Autodesk Inventor part; units mm, degrees
ref_plane "a1_XY" through (0, 8.636, -14.224) normal (0, 1, 0) x (1, 0, 0)
ref_plane "a1_YZ" through (0, 8.636, -14.224) normal (1, 0, 0) x (0, 0, -1)
ref_plane "a1_ZX" through (0, 8.636, -14.224) normal (0, 0, -1) x (0, 1, 0)
sketch "Sketch_1" plane through (0, 0, 0) normal (0, 0, 1) x (1, 0, 0)
  line L0 (0, 0) -> (0, 8.636)
  line L1 (0, 8.636) -> (14.224, 8.636)
  line L2 (14.224, 8.636) -> (14.224, 0)
  line L3 (14.224, 0) -> (0, 0)
  line L4 (0, 0) -> (0, 8.636)
revolve "Revolution1" add sketch "Sketch_1" angle 360 about axis through (0, 0, 0) along (0, -1, 0)
sketch "Sketch_37" plane through (0, 0, 0) normal (0, 0, 1) x (1, 0, 0)
  line L0 (-5.9667, 5.08) -> (-14.224, 5.08)
  line L1 (-14.224, 5.08) -> (-14.224, 9.0488)
  line L2 (-14.224, 9.0488) -> (-13.716, 9.0488)
  line L3 (-13.716, 9.0488) -> (-13.716, 7.493)
  line L4 (-13.716, 7.493) -> (-13.2867, 7.0637)
  line L5 (-13.2867, 7.0637) -> (-7.112, 7.0637)
  line L6 (-7.112, 7.0637) -> (-5.9667, 5.08)
  line L7 (-5.9667, 5.08) -> (-14.224, 5.08)
revolve "Revolution2" cut sketch "Sketch_37" angle 360 about axis through (-5.9667, 5.08, 0) along (1, 0, 0)
thread "Thread1"
sketch "Sketch3" plane through (0, 0, 0) normal (0, -1, 0) x (1, 0, 0)
  point P0 (0, 0)
hole "Hole1" at (0, 0, 0) direction (0, 1, 0) diameter 6.4008 depth 8.636
sketch "Sketch_9" plane through (0, 0, 0) normal (0, 0, 1) x (1, 0, 0)
  line L0 (0, 0) -> (0, 2.54)
  line L1 (0, 2.54) -> (7.747, 2.54)
  line L2 (7.747, 2.54) -> (7.747, 0)
  line L3 (7.747, 0) -> (0, 0)
  line L4 (0, 0) -> (0, 2.54)
revolve "Revolution3" cut sketch "Sketch_9" angle 360 about axis through (0, 0, 0) along (0, -1, 0)
sketch "Sketch5" plane through (0, 8.636, 0) normal (0, 1, 0) x (1, 0, 0)
  point P0 (0, -11.176)
hole "Hole2" at (0, 8.636, 11.176) direction (0, -1, 0) diameter 3.048 depth 8.636 counterbore diameter 4.7752 counterbore depth 3.048
sketch "Sketch6" plane through (0, 8.636, 0) normal (0, 1, 0) x (1, 0, 0)
  point P0 (0, 11.176)
hole "Hole3" at (0, 8.636, -11.176) direction (0, -1, 0) diameter 3.048 depth 8.636 counterbore diameter 4.7752 counterbore depth 3.048
sketch "Sketch7" plane through (0, 0, 0) normal (0, -1, 0) x (1, 0, 0)
  point P0 (-7.9026, 7.9026)
hole "Hole4" at (-7.9026, 0, 7.9026) direction (0, 1, 0) diameter 3.048 depth 2.54
sketch "Sketch8" plane through (0, 0, 0) normal (0, -1, 0) x (1, 0, 0)
  point P0 (7.9026, 7.9026)
hole "Hole5" at (7.9026, 0, 7.9026) direction (0, 1, 0) diameter 3.048 depth 2.54
sketch "Sketch9" plane through (0, 0, 0) normal (0, -1, 0) x (1, 0, 0)
  point P0 (7.9026, -7.9026)
hole "Hole6" at (7.9026, 0, -7.9026) direction (0, 1, 0) diameter 3.048 depth 2.54
sketch "Sketch10" plane through (0, 0, 0) normal (0, -1, 0) x (1, 0, 0)
  point P0 (-7.9026, -7.9026)
hole "Hole7" at (-7.9026, 0, -7.9026) direction (0, 1, 0) diameter 3.048 depth 2.54
ref_plane "a1_XY" through (0, 8.636, -14.224) normal (0, 1, 0) x (1, 0, 0)
ref_plane "a1_YZ" through (0, 8.636, -14.224) normal (1, 0, 0) x (0, 0, -1)
ref_plane "a1_ZX" through (0, 8.636, -14.224) normal (0, 0, -1) x (0, 1, 0)
ref_plane "a2_XY" through (0, 8.636, 14.224) normal (0, 1, 0) x (1, 0, 0)
ref_plane "a2_YZ" through (0, 8.636, 14.224) normal (1, 0, 0) x (0, 0, -1)
ref_plane "a2_ZX" through (0, 8.636, 14.224) normal (0, 0, -1) x (0, 1, 0)
ref_plane "ar3_XY" through (-7.9026, 2.54, 7.9026) normal (0, 1, 0) x (1, 0, 0)
ref_plane "ar3_YZ" through (-7.9026, 2.54, 7.9026) normal (1, 0, 0) x (0, 0, -1)
ref_plane "ar3_ZX" through (-7.9026, 2.54, 7.9026) normal (0, 0, -1) x (0, 1, 0)
ref_plane "ar4_XY" through (7.9026, 2.54, 7.9026) normal (0, 1, 0) x (1, 0, 0)
ref_plane "ar4_YZ" through (7.9026, 2.54, 7.9026) normal (1, 0, 0) x (0, 0, -1)
ref_plane "ar4_ZX" through (7.9026, 2.54, 7.9026) normal (0, 0, -1) x (0, 1, 0)
ref_plane "ar5_XY" through (7.9026, 2.54, -7.9026) normal (0, 1, 0) x (1, 0, 0)
ref_plane "ar5_YZ" through (7.9026, 2.54, -7.9026) normal (1, 0, 0) x (0, 0, -1)
ref_plane "ar5_ZX" through (7.9026, 2.54, -7.9026) normal (0, 0, -1) x (0, 1, 0)
ref_plane "ar6_XY" through (-7.9026, 2.54, -7.9026) normal (0, 1, 0) x (1, 0, 0)
ref_plane "ar6_YZ" through (-7.9026, 2.54, -7.9026) normal (1, 0, 0) x (0, 0, -1)
ref_plane "ar6_ZX" through (-7.9026, 2.54, -7.9026) normal (0, 0, -1) x (0, 1, 0)
ref_plane "b1_XY" through (0, 8.636, 0) normal (0, 1, 0) x (1, 0, 0)
ref_plane "b1_YZ" through (0, 8.636, 0) normal (1, 0, 0) x (0, 0, -1)
ref_plane "b1_ZX" through (0, 8.636, 0) normal (0, 0, -1) x (0, 1, 0)
ref_plane "c1_XY" through (0, 8.636, -11.176) normal (0, 1, 0) x (1, 0, 0)
ref_plane "c1_YZ" through (0, 8.636, -11.176) normal (1, 0, 0) x (0, 0, -1)
ref_plane "c1_ZX" through (0, 8.636, -11.176) normal (0, 0, -1) x (0, 1, 0)
ref_plane "c2_XY" through (0, 8.636, 11.176) normal (0, 1, 0) x (1, 0, 0)
ref_plane "c2_YZ" through (0, 8.636, 11.176) normal (1, 0, 0) x (0, 0, -1)
ref_plane "c2_ZX" through (0, 8.636, 11.176) normal (0, 0, -1) x (0, 1, 0)
ref_plane "d1_XY" through (-1.524, 8.636, -11.176) normal (0, 1, 0) x (1, 0, 0)
ref_plane "d1_YZ" through (-1.524, 8.636, -11.176) normal (1, 0, 0) x (0, 0, -1)
ref_plane "d1_ZX" through (-1.524, 8.636, -11.176) normal (0, 0, -1) x (0, 1, 0)
ref_plane "d2_XY" through (1.524, 8.636, -11.176) normal (0, 1, 0) x (1, 0, 0)
ref_plane "d2_YZ" through (1.524, 8.636, -11.176) normal (1, 0, 0) x (0, 0, -1)
ref_plane "d2_ZX" through (1.524, 8.636, -11.176) normal (0, 0, -1) x (0, 1, 0)
ref_plane "j_XY" through (0, 0, 0) normal (0, 1, 0) x (1, 0, 0)
ref_plane "j_YZ" through (0, 0, 0) normal (1, 0, 0) x (0, 0, -1)
ref_plane "j_ZX" through (0, 0, 0) normal (0, 0, -1) x (0, 1, 0)
ref_plane "k1_XY" through (-14.224, 5.08, 0) normal (0, 0, 1) x (1, 0, 0)
ref_plane "k1_YZ" through (-14.224, 5.08, 0) normal (1, 0, 0) x (0, 1, 0)
ref_plane "k1_ZX" through (-14.224, 5.08, 0) normal (0, 1, 0) x (0, 0, 1)
ref_plane "k2_XY" through (-14.224, 8.636, 0) normal (0, 0, 1) x (1, 0, 0)
ref_plane "k2_YZ" through (-14.224, 8.636, 0) normal (1, 0, 0) x (0, 1, 0)
ref_plane "k2_ZX" through (-14.224, 8.636, 0) normal (0, 1, 0) x (0, 0, 1)
ref_plane "l1_XY" through (-14.224, 7.493, 0) normal (0, 0, 1) x (1, 0, 0)
ref_plane "l1_YZ" through (-14.224, 7.493, 0) normal (1, 0, 0) x (0, 1, 0)
ref_plane "l1_ZX" through (-14.224, 7.493, 0) normal (0, 1, 0) x (0, 0, 1)
ref_plane "l2_XY" through (-14.224, 2.667, 0) normal (0, 0, 1) x (1, 0, 0)
ref_plane "l2_YZ" through (-14.224, 2.667, 0) normal (1, 0, 0) x (0, 1, 0)
ref_plane "l2_ZX" through (-14.224, 2.667, 0) normal (0, 1, 0) x (0, 0, 1)
ref_plane "rg_XY" through (0, 8.636, 0) normal (0, 1, 0) x (1, 0, 0)
ref_plane "rg_YZ" through (0, 8.636, 0) normal (1, 0, 0) x (0, 0, -1)
ref_plane "rg_ZX" through (0, 8.636, 0) normal (0, 0, -1) x (0, 1, 0)
ref_plane "rh_XY" through (0, 8.636, 0) normal (0, 1, 0) x (1, 0, 0)
ref_plane "rh_YZ" through (0, 8.636, 0) normal (1, 0, 0) x (0, 0, -1)
ref_plane "rh_ZX" through (0, 8.636, 0) normal (0, 0, -1) x (0, 1, 0)
ref_plane "to_dummy_XY" through (0, 8.636, 0) normal (0, 1, 0) x (1, 0, 0)
ref_plane "to_dummy_YZ" through (0, 8.636, 0) normal (1, 0, 0) x (0, 0, -1)
ref_plane "to_dummy_ZX" through (0, 8.636, 0) normal (0, 0, -1) x (0, 1, 0)
ref_plane "to_nut_XY" through (0, 10.16, 0) normal (0, 1, 0) x (1, 0, 0)
ref_plane "to_nut_YZ" through (0, 10.16, 0) normal (1, 0, 0) x (0, 0, -1)
ref_plane "to_nut_ZX" through (0, 10.16, 0) normal (0, 0, -1) x (0, 1, 0)
ref_plane "to_rod_XY" through (0, 8.636, 0) normal (0, 1, 0) x (1, 0, 0)
ref_plane "to_rod_YZ" through (0, 8.636, 0) normal (1, 0, 0) x (0, 0, -1)
ref_plane "to_rod_ZX" through (0, 8.636, 0) normal (0, 0, -1) x (0, 1, 0)
ref_plane "to_tube_XY" through (0, 2.54, 0) normal (0, 1, 0) x (1, 0, 0)
ref_plane "to_tube_YZ" through (0, 2.54, 0) normal (1, 0, 0) x (0, 0, -1)
ref_plane "to_tube_ZX" through (0, 2.54, 0) normal (0, 0, -1) x (0, 1, 0)
ref_plane "to_wiper_XY" through (0, 8.636, 0) normal (0, 1, 0) x (1, 0, 0)
ref_plane "to_wiper_YZ" through (0, 8.636, 0) normal (1, 0, 0) x (0, 0, -1)
ref_plane "to_wiper_ZX" through (0, 8.636, 0) normal (0, 0, -1) x (0, 1, 0)
ref_plane "track1_XY" through (-7.874, 0, 0) normal (0, 1, 0) x (1, 0, 0)
ref_plane "track1_YZ" through (-7.874, 0, 0) normal (1, 0, 0) x (0, 0, -1)
ref_plane "track1_ZX" through (-7.874, 0, 0) normal (0, 0, -1) x (0, 1, 0)
ref_plane "track2_XY" through (0, 0, -7.874) normal (0, 1, 0) x (1, 0, 0)
ref_plane "track2_YZ" through (0, 0, -7.874) normal (1, 0, 0) x (0, 0, -1)
ref_plane "track2_ZX" through (0, 0, -7.874) normal (0, 0, -1) x (0, 1, 0)
ref_plane "track3_XY" through (7.874, 0, 0) normal (0, 1, 0) x (1, 0, 0)
ref_plane "track3_YZ" through (7.874, 0, 0) normal (1, 0, 0) x (0, 0, -1)
ref_plane "track3_ZX" through (7.874, 0, 0) normal (0, 0, -1) x (0, 1, 0)
ref_plane "track4_XY" through (0, 0, 7.874) normal (0, 1, 0) x (1, 0, 0)
ref_plane "track4_YZ" through (0, 0, 7.874) normal (1, 0, 0) x (0, 0, -1)
ref_plane "track4_ZX" through (0, 0, 7.874) normal (0, 0, -1) x (0, 1, 0)
properties part number "02-1-0.13-FO1_BM_heads" material "Steel"
Model file for the job. Use its own axes, mm. A direction names the side the tool comes from. Coordinates: 2 decimals unless noted, no trailing zeros. Write each loop counter-clockwise with the first axis right and the second up, starting at its lowest first coordinate (ties: lowest second). Pieces come first, ordered by that corner, then holes. Notation, with made-up numbers: (47, 47.5) - (105, 47.5) arc R19 ccw to (105, 57.5) - close; hole circle Ø3 at (25.5, 32.5). An arc over 180 degrees is marked (long way). One line per item, written item: value. Start each with the question number.
1. Flat gauge pins, fed straight in: pin 1 (0.9 mm diameter, centred on x = 7.5, z = 7.5, fed in from -Y); pin 2 (2.5 mm diameter, centred on x = -7.5, z = 8, fed in from -Y); pin 3 (3 mm diameter, centred on y = 5.5, z = 8.5, fed in from -X); pin 4 (1.5 mm diameter, centred on y = 4, z = -3.5, fed in from -X). Where does each tip first touch, or does it go through?
2. Mould opens along Y. For faces 4 (the flat face through (-8, 2.54, 8)), 5 (the cylindrical face through (-10.16, 6.97, 0.6)), 6 (the cylindrical face through (-0.07, 2.75, -12.7)) say: released by +Y, released by -Y, zero draft, split by the parting line, or undercut.
3. Slice it at B-B (y = 2). Write the cut outline in (x, z).
4. Slice it at A-A (x = 0). Write the cut outline in (y, z).
5. Tool access for faces 1 (the cylindrical face through (1.95, 5.63, 2.54)), 2 (the cylindrical face through (-0.1, 7.09, 8.79)), 3 (the cylindrical face through (8.49, 1.29, -9.31)): list every direction of +Z, -Z, +X, -X, +Y, -Y with a clear straight run to the whole face (end or side of a thin tool).
6. Slice it at C-C (z = -11.5). Write the cut outline in (x, y).
7. Probe line 1 (Z direction, x = 0, y = 7.2); line 2 (X direction, y = 2, z = -6.75); line 3 (X direction, y = 2, z = -8). List the from-to ranges inside material, lowest first. Write a range as from..to.
8. Slice it at D-D (z = -7.25). Write the cut outline in (x, y).
Answers below:
1. pin 1: stops at y = 2.54
1. pin 2: stops at y = 0
1. pin 3: stops at x = -12.38
1. pin 4: stops at x = -13.78
2. face 4: released by -Y
2. face 5: undercut
2. face 6: zero draft
3. outline: (-14, -2.5) arc R14.22 ccw (long way) to (-14, 2.5) - (-13.72, 2.5) - (-13.72, -2.5) - close; hole circle Ø3.05 at (-7.9, -7.9); hole circle Ø3.05 at (-7.9, 7.9); hole circle Ø15.49 at (0, 0); hole circle Ø3.05 at (0, -11.18); hole circle Ø3.05 at (0, 11.18); hole circle Ø3.05 at (7.9, -7.9); hole circle Ø3.05 at (7.9, 7.9)
4. outline: (0, -14.22) - (8.64, -14.22) - (8.64, -13.56) - (5.59, -13.56) - (5.59, -12.7) - (0, -12.7) - close; (0, -9.65) - (5.59, -9.65) - (5.59, -8.79) - (8.64, -8.79) - (8.64, -3.2) - (2.54, -3.2) - (2.54, -7.75) - (0, -7.75) - close; (0, 7.75) - (2.54, 7.75) - (2.54, 3.2) - (8.64, 3.2) - (8.64, 8.79) - (5.59, 8.79) - (5.59, 9.65) - (0, 9.65) - close; (0, 12.7) - (5.59, 12.7) - (5.59, 13.56) - (8.64, 13.56) - (8.64, 14.22) - (0, 14.22) - close
5. face 1: +Y, -Y
5. face 2: +Y
5. face 3: -Y
6. outline: (-8.37, 0) - (-1.49, 0) - (-1.49, 5.59) - (-2.37, 5.59) - (-2.37, 8.64) - (-8.37, 8.64) - close; (1.49, 0) - (8.37, 0) - (8.37, 8.64) - (2.37, 8.64) - (2.37, 5.59) - (1.49, 5.59) - close
7. line 1: z = -14.22..-13.56, -8.79..-3.2, 3.2..8.79, 13.56..14.22
7. line 2: x = -12.52..-8.9, -6.91..-3.8, 3.8..6.91, 8.9..12.52
7. line 3: x = -11.76..-9.42, -6.38..6.38, 9.42..11.76
8. outline: (-12.24, 0) - (-9.28, 0) - (-9.28, 2.54) - (-6.53, 2.54) - (-6.53, 0) - (-2.73, 0) - (-2.73, 2.54) - (2.73, 2.54) - (2.73, 0) - (6.53, 0) - (6.53, 2.54) - (9.28, 2.54) - (9.28, 0) - (12.24, 0) - (12.24, 8.64) - (-12.24, 8.64) - close
